from build123d import *

# Parameters (mm, degrees)
EXTRUDE_1_DEPTH          = 1
SKETCH_2_OUTSIDE_W       = 20.56
SKETCH_2_OUTSIDE_H       = 19.785
SKETCH_2_OUTSIDE_R       = 2.605451242
CUT_EXTRUDE_1_DEPTH      = 5.459704035
CUT_EXTRUDE_1_DRAFT      = -45
MIRROR_1_COPY_1_SKETCH_W = 20.56
MIRROR_1_COPY_1_SKETCH_H = 19.785
MIRROR_1_COPY_1_SKETCH_R = 2.605451242
MIRROR_1_COPY_1_DEPTH    = 5.459704035
MIRROR_1_COPY_1_DRAFT    = -45


with BuildPart() as part:
    # 草图1 → 凸台-拉伸1 (new, symmetric)
    with BuildSketch(Plane(origin=(0, 0, 0), x_dir=(1, 0, 0), z_dir=(0, 1, 0))):
        Polygon((-1.520889796, -2.576331008), (1.479110204, -2.605355672), (3.0042463, -0.021791793), (1.529382397, 2.59079675), (-1.470617603, 2.619821415), (-2.9957537, 0.036257535), align=None)
    extrude(amount=EXTRUDE_1_DEPTH, both=True)


with BuildPart() as cut_extrude_1_tool:
    # 草图2 outside → 切除-拉伸1 (with draft: the straight prism first)
    with BuildSketch(Plane(origin=(0, 1, 0), x_dir=(1, 0, 0), z_dir=(0, 1, 0))):
        with Locations((0.004, 0.0075)):
            Rectangle(SKETCH_2_OUTSIDE_W, SKETCH_2_OUTSIDE_H)
        Circle(SKETCH_2_OUTSIDE_R, mode=Mode.SUBTRACT)
    extrude(amount=-CUT_EXTRUDE_1_DEPTH)
    # 切除-拉伸1: the draft: its side faces are tilted about the plane it starts from
    cut_extrude_1_sides = [cut_extrude_1_tool.faces().sort_by_distance(p)[0] for p in [
        (0.004, -1.729852017, 9.885),
        (10.284, -1.729852017, -0.0075),
        (0.004, -1.729852017, -9.9),
        (-10.276, -1.729852017, -0.0075),
        (-2.605451242, -1.729852017, 0),
    ]]
    draft(cut_extrude_1_sides, Plane(origin=(0, 1, 0), x_dir=(1, 0, 0), z_dir=(0, 1, 0)), CUT_EXTRUDE_1_DRAFT)


with BuildPart() as part_1:
    add(part.part)

    # 切除-拉伸1: cut by cut_extrude_1_tool
    add(cut_extrude_1_tool.part, mode=Mode.SUBTRACT)


with BuildPart() as mirror_1_copy_1_tool:
    # 镜向1 copy 1 sketch → 镜向1 copy 1 (with draft: the straight prism first)
    with BuildSketch(Plane.XZ.offset(1)):
        with Locations((0.004, -0.0075)):
            Rectangle(MIRROR_1_COPY_1_SKETCH_W, MIRROR_1_COPY_1_SKETCH_H)
        Circle(MIRROR_1_COPY_1_SKETCH_R, mode=Mode.SUBTRACT)
    extrude(amount=-MIRROR_1_COPY_1_DEPTH)
    # 镜向1 copy 1: the draft: its side faces are tilted about the plane it starts from
    mirror_1_copy_1_sides = [mirror_1_copy_1_tool.faces().sort_by_distance(p)[0] for p in [
        (0.004, 1.729852017, 9.885),
        (10.284, 1.729852017, -0.0075),
        (0.004, 1.729852017, -9.9),
        (-10.276, 1.729852017, -0.0075),
        (-2.605451242, 1.729852017, 0),
    ]]
    draft(mirror_1_copy_1_sides, Plane.XZ.offset(1), MIRROR_1_COPY_1_DRAFT)


with BuildPart() as part_2:
    add(part_1.part)

    # 镜向1 copy 1: cut by mirror_1_copy_1_tool
    add(mirror_1_copy_1_tool.part, mode=Mode.SUBTRACT)


solid = part_2.part
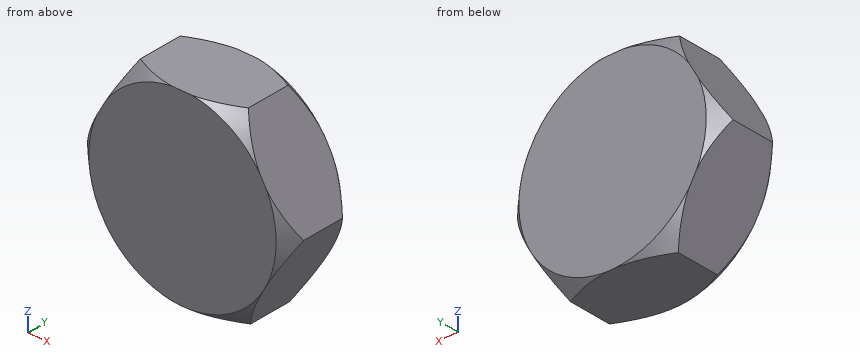
Verification items for the finished model (mm, model axes). Round coordinates to 2 decimals unless told otherwise and drop trailing zeros. Loops run counter-clockwise (first coordinate to the right, second up) from the corner with the lowest first, then second, coordinate; pieces in that order, holes last. Notation, with made-up numbers: (60.25, 62) - (75.25, 62) arc R7 ccw to (75.25, 69) - close; hole circle Ø1 at (-8.75, 69.5). An arc over 180 degrees is marked (long way). Answer in a Markdown table with one row per item. Add a question column.
Q1. Section check A-A on y = 0.8. Enter the section's corners in (x, z), plus the area to 3 significant figures.
Q2. Gauge pin test, flat ends, axial feed: pin 1 (1.5 mm diameter, centred on x = 2, z = -2, fed in from +Y); pin 2 (1 mm diameter, centred on y = -0.5, z = -2, fed in from +X). Record the tip position at first contact, or that the pin passes through.
Q3. Section check B-B on y = -0.1. Enter the section's corners in (x, z).
Q4. Material ranges on line 1 (Z direction, x = -0.25, y = 0.6); line 2 (X direction, y = -0.35, z = -0.1); line 3 (Z direction, x = -2, y = 0.55), recorded low to high.
Found:
| question | item | result |
|---|---|---|
| 1 | outline | (-2.79, 0.34) arc R2.81 ccw to (-2.78, -0.41) - (-1.7, -2.23) arc R2.81 ccw to (-1.01, -2.62) - (1.07, -2.6) arc R2.81 ccw to (1.76, -2.19) - (2.78, -0.37) arc R2.81 ccw to (2.78, 0.41) - (1.7, 2.23) arc R2.81 ccw to (1.05, 2.6) - (-1.1, 2.58) arc R2.81 ccw to (-1.73, 2.21) - close |
| 1 | area | 23.0 mm² |
| 2 | pin 1 | stops at y = 1 |
| 2 | pin 2 | stops at x = 2.15 |
| 3 | outline | (-3, -0.04) - (-1.47, -2.62) - (1.53, -2.59) - (3, 0.02) - (1.48, 2.61) - (-1.52, 2.58) - close |
| 4 | line 1 | z = -2.61 to 2.59 |
| 4 | line 2 | x = -2.96 to 2.94 |
| 4 | line 3 | z = -1.72 to 1.73 |
